Part model, mm, in its own coordinate system. A direction names the side the tool comes from. Coordinates: 2 decimals unless noted, no trailing zeros. Order: outer loops, then holes, each group sorted by start corner. A loop starts at its lowest first (then second) coordinate and runs counter-clockwise, first axis right, second up. Notation, with made-up numbers: (42.25, -19.5) - (49.25, -19.5) arc R20 cw to (49.25, -3.5) - close; hole circle Ø2 at (-6, -10.5). An arc over 180 degrees is marked (long way). Use a Markdown table: item, result. Add a question column.
1) Saw through at A-A on z = 9. List the corners of the cut face in (x, y) (3 decimals).
2) Saw through at C-C on x = -78.5. List the corners of the cut face in (y, z).
3) Saw through at B-B on y = 90. List the corners of the cut face in (x, z).
4) Drop flat-ended pins along their axis: P1, Ø1.5, axis at y = 65, z = 9.5, coming from the +X side; P2, Ø4, axis at x = -117, z = 11.5, coming from the +Y side; P3, Ø4, axis at x = -132.07, y = 175.82, coming from the -Z side; P4, Ø2, axis at x = -92.5, z = 2, coming from the -Y side. Give the stop position or say it passes through.
5) Tool access for faces 1 (the face through (-114, 31, 12.7)), 2 (the face through (-106.672, 99, 6)): list every direction of +Z, -Z, +X, -X, +Y, -Y with a clear straight run to the whole face (end or side of a thin tool).
6) Two-plate mould, pull along Y, no slides. Class faces 3 (the face through (-132.631, 201.214, 6.261)), 4 (the face through (1, -116.28, 6)), 5 (the face through (-132.486, 172.672, 6.261)): +Y half, -Y half, draft (parallel to the pull), parting line (faces both ways), or undercut.
7) Wall check: L1, parallel to X at y = 97.5, z = 7.25; L2, parallel to Y at x = 17, z = 6; L3, parallel to Y at x = 8, z = 6.75. Give the ranges that are in metal, low to high. Write a range as [from, to].
Autodesk Inventor part; units mm, degrees
ref_plane "YZ Plane" through (0, 0, 0) normal (1, 0, 0) x (0, 1, 0)
ref_plane "XZ Plane" through (0, 0, 0) normal (0, 1, 0) x (-1, 0, 0)
ref_plane "XY Plane" through (0, 0, 0) normal (0, 0, 1) x (1, 0, 0)
sketch "Sketch1" plane through (0, 0, 0) normal (0, 0, 1) x (1, 0, 0)
  circle A0 centre (-132.0723, 175.8198) radius 3.175
  arc A1 (-106.6723, 175.8198) -> (-157.4723, 175.8198) centre (-132.0723, 175.8198) ccw
  arc A2 (-106.6723, 23.4198) -> (20.3277, -103.5802) centre (20.3277, 23.4198) ccw
  arc A3 (-157.4723, 23.4198) -> (-17.7723, -116.2802) centre (-17.7723, 23.4198) ccw
  line L0 (-157.4723, 175.8198) -> (-157.4723, 23.4198)
  line L1 (-106.6723, 23.4198) -> (-106.6723, 175.8198)
  line L2 (-17.7723, -116.2802) -> (20.3277, -116.2802)
  arc A4 (20.3277, -116.2802) -> (20.3277, -103.5802) centre (20.3277, -109.9302) ccw
  dimension "d23" = 6.35
  dimension "d24" = 50.8
  dimension "d25" = 25.4
  dimension "d26" = 127
  dimension "d27" = 139.7
  dimension "d28" = 152.4
  dimension "d29" = 152.4
  dimension "d30" = 6.35
  dimension "d31" = 38.1
extrude "Extrusion2" add sketch "Sketch1" along normal blind 12.7
properties part number "Bottom IntakeBar"
Results are:
| question | item | result |
|---|---|---|
| 1 | outline | (-157.472, 23.42) arc R139.7 ccw to (-17.772, -116.28) - (20.328, -116.28) arc R6.35 ccw to (20.328, -103.58) arc R127 cw to (-106.672, 23.42) - (-106.672, 175.82) arc R25.4 ccw to (-157.472, 175.82) - close; hole circle Ø6.35 at (-132.072, 175.82) |
| 2 | outline | (-102.39, 0) - (-56.34, 0) - (-56.34, 12.7) - (-102.39, 12.7) - close |
| 3 | outline | (-157.47, 0) - (-106.67, 0) - (-106.67, 12.7) - (-157.47, 12.7) - close |
| 4 | P1 | x = -106.67 |
| 4 | P2 | y = 197.6 |
| 4 | P3 | through |
| 4 | P4 | y = -95.24 |
| 5 | face 1 | +Z, +X, -X, +Y, -Y |
| 5 | face 2 | +Z, -Z, +X, +Y |
| 6 | face 3 | +Y half |
| 6 | face 4 | -Y half |
| 6 | face 5 | undercut |
| 7 | L1 | [-157.47, -106.67] |
| 7 | L2 | [-116.28, -103.54] |
| 7 | L3 | [-116.28, -102.98] |
